from build123d import *

# Parameters (mm, degrees)
SKETCH1_R           = 3.95
BOSS_EXTRUDE1_DEPTH = 30
SKETCH2_R           = 5.2
BOSS_EXTRUDE2_DEPTH = 2
SKETCH5_W           = 2
SKETCH5_H           = 2.467717667
BOSS_EXTRUDE3_DEPTH = 19
SKETCH6_R           = 9.177685327
CUT_EXTRUDE1_DEPTH  = 0.321276311
SKETCH8_W           = 2.5
SKETCH8_H           = 2
BOSS_EXTRUDE4_DEPTH = 8


with BuildPart() as part:
    # Sketch1 → Boss-Extrude1 (new body)
    with BuildSketch(Plane(origin=(0, 0, 0), x_dir=(1, 0, 0), z_dir=(0, 1, 0))):
        with Locations(Location((0, 0, 0), (0, 0, 270))):
            Circle(SKETCH1_R)
    extrude(amount=BOSS_EXTRUDE1_DEPTH)

    # Sketch2 → Boss-Extrude2 (add)
    with BuildSketch(Plane.XZ):
        with Locations(Location((0, 0, 0), (0, 0, 270))):
            Circle(SKETCH2_R)
    extrude(amount=BOSS_EXTRUDE2_DEPTH)

    # Sketch5 → Boss-Extrude3 (add)
    with BuildSketch(Plane(origin=(0, 0, 0), x_dir=(0, 0, -1), z_dir=(1, 0, 0))):
        with Locations((0, 29.087417478)):
            Rectangle(SKETCH5_W, SKETCH5_H)
    extrude(amount=BOSS_EXTRUDE3_DEPTH)

    # Sketch6 → Cut-Extrude1 (cut)
    with BuildSketch(Plane(origin=(0, 30, 0), x_dir=(1, 0, 0), z_dir=(0, 1, 0))):
        Circle(SKETCH6_R)
    extrude(amount=CUT_EXTRUDE1_DEPTH, mode=Mode.SUBTRACT)

    # Sketch8 → Boss-Extrude4 (add)
    with BuildSketch(Plane.XY):
        with Locations((0, -1)):
            Rectangle(SKETCH8_W, SKETCH8_H)
    extrude(amount=BOSS_EXTRUDE4_DEPTH)


solid = part.part
Read the model definition and answer for the solid it produces. Units are mm, in the model's axes. A direction names the side the tool comes from. Round coordinates to 2 decimals unless told otherwise and drop trailing zeros. Write each loop counter-clockwise with the first axis right and the second up, starting at its lowest first coordinate (ties: lowest second). Pieces come first, ordered by that corner, then holes.
1. The part is cut by section B-B, the plane z = 0. Determine the outline of the cut face in (x, y), then the cut area to 3 significant figures.
2. The part is cut by section A-A, the plane x = 0. Determine the outline of the cut face in (y, z), then the cut area to 3 significant figures.
3. The part is cut by section D-D, the plane x = 16.5. Determine the outline of the cut face in (y, z).
4. Which of the six approach directions +Z, -Z, +X, -X, +Y, -Y give full straight-line access (tool end or side, diameter ignored) to faces 1 (the face through (1, 30, 0)), 2 (the face through (-1.25, -1, 7)), 3 (the face through (1.25, -1, 7))?
5. Straight lines are drawn through the part: L1, parallel to Y at x = 1.5, z = 0.75; L2, parallel to Z at x = -0.25, y = 5.5; L3, parallel to Z at x = -3.5, y = 26. For each, find the intervals that lie inside material, in ascending order.
6. Given pin 1 Ø6.5 at (x, z) = (2.5, -1.5) entering from +Y; pin 2 Ø0.6 at (y, z) = (-1, 7) entering from -X; pin 3 Ø1 at (x, z) = (8.5, 0.5) entering from -Y, each flat-ended and moving along its own axis, determine where each tip first touches the part or whether it passes through.
7. The part is cut by section C-C, the plane y = 15. Determine the outline of the cut face in (x, z).
Values:
1. outline: (-5.2, -2) - (5.2, -2) - (5.2, 0) - (3.95, 0) - (3.95, 27.85) - (19, 27.85) - (19, 30.32) - (9.18, 30.32) - (9.18, 30) - (-3.95, 30) - (-3.95, 0) - (-5.2, 0) - close
1. area: 293 mm2
2. outline: (-2, -5.2) - (0, -5.2) - (0, -3.95) - (30, -3.95) - (30, 3.95) - (0, 3.95) - (0, 8) - (-2, 8) - close
2. area: 263 mm2
3. outline: (27.85, -1) - (30.32, -1) - (30.32, 1) - (27.85, 1) - close
4. face 1: +Z, -Z, -X, +Y
4. face 2: +Z, -X, +Y, -Y
4. face 3: +Z, +X, +Y, -Y
5. L1: y = -2 to 30
5. L2: z = -3.94 to 3.94
5. L3: z = -1.83 to 1.83
6. pin 1: stops at y = 30
6. pin 2: stops at x = -1.25
6. pin 3: stops at y = 27.85
7. outline: circle Ø7.9 at (0, 0)
